from build123d import *

# Parameters (mm, degrees)
F0_W           = 838.2
F0_H           = 50.8
F1_DEPTH       = 76.2
F3_T           = -8.89
F4_D           = 12.7
F4_CSINK_D     = 20.32
F4_CSINK_ANGLE = 90
F5_R           = 5.08


with BuildPart() as f1:
    # F0 (on Front) → F1 (new body)
    with BuildSketch(Plane.XZ):
        with Locations((419.1, -25.4)):
            Rectangle(F0_W, F0_H)
    extrude(amount=F1_DEPTH)

    # F3
    f3_openings = [f1.faces().sort_by_distance(p)[0] for p in [
        (838.2, -38.1, -25.4),
        (419.1, -38.1, -50.8),
        (0, -38.1, -25.4),
    ]]
    offset(amount=F3_T, openings=f3_openings)

    # F4 (through all)
    with Locations(Plane.XZ.offset(76.2)):
        with Locations((38.1, -29.845), (800.1, -29.845)):
            CounterSinkHole(F4_D / 2, F4_CSINK_D / 2, counter_sink_angle=F4_CSINK_ANGLE)

    # F5
    f5_edges = [f1.edges().sort_by_distance(p)[0] for p in [
        (419.1, -76.2, 0),
        (419.1, 0, 0),
    ]]
    fillet(f5_edges, radius=F5_R)


solid = f1.part
Geometry: final body of the model. Coordinates: model frame, mm. A direction names the side the tool comes from. Give positions to 0.01 mm unless a question says otherwise; leave off trailing zeros. Loops run counter-clockwise (first coordinate to the right, second up) from the corner with the lowest first, then second, coordinate; pieces in that order, holes last. Notation, with made-up numbers: (73, -24.75) - (105, -24.75) arc R14 ccw to (105, 1.25) - close; hole circle Ø9 at (85.25, -38.5). An arc over 180 degrees is marked (long way). One line per question, with ' | ' between items. Start each with the question number.
(1) Contact query for flat-ended pins moving along their axis: pin 1 (3 mm diameter, centred on x = 671, y = -39.5, fed in from -Z); pin 2 (14.5 mm diameter, centred on x = 800.1, z = -29.845, fed in from -Y); pin 3 (16.5 mm diameter, centred on x = 800.1, z = -29.845, fed in from -Y). Output: stop coordinate, or through.
(2) Pull-direction query (X, two-part tool) for faces 3 (the flat face through (838.2, -38, -3)), 4 (the flat face through (413, -38, -8.89)), 5 (the cylindrical face through (38.93, -69.81, -23.55)), 6 (the flat face through (0, -38, -3)); classes: released by +X, released by -X, zero draft, split by the parting line, or undercut.
(3) Section query A-A on x = 776. Return loops of the section in (y, z), then the cut area to 3 significant figures.
(4) Reachability of faces 1 (the flat face through (413, -76.2, -28)), 2 (the flat face through (413, -8.89, -30)) from +Z, -Z, +X, -X, +Y, -Y: full face, straight path, thin tool, end or side. Return the list, or none.
(5) Section query B-B on y = -40. Return loops of the section in (x, z).
(6) Ray query, line 1 (Y direction, x = 182, z = -44); line 2 (X direction, y = -68, z = -27); line 3 (X direction, y = -71, z = -27.5). Return the intervals inside material, ascending. Write a range as from..to.
The answers:
1) pin 1: z = -8.89 | pin 2: y = -73.29 | pin 3: y = -74.29
2) face 3: released by +X | face 4: zero draft | face 5: undercut | face 6: released by -X
3) outline: (-76.2, -50.8) - (-67.31, -50.8) - (-67.31, -8.89) - (-8.89, -8.89) - (-8.89, -50.8) - (0, -50.8) - (0, -5.08) arc R5.08 ccw to (-5.08, 0) - (-71.12, 0) arc R5.08 ccw to (-76.2, -5.08) - close | area: 1,410 mm2
4) face 1: +Z, -Z, +X, -X, -Y | face 2: -Z, +X, -X
5) outline: (0, -8.89) - (838.2, -8.89) - (838.2, 0) - (0, 0) - close
6) line 1: -76.2..-67.31, -8.89..0 | line 2: 0..32.42, 43.78..794.42, 805.78..838.2 | line 3: 0..32.2, 44..794.2, 806..838.2
